Part model, mm, in its own coordinate system. Coordinates: 2 decimals unless noted, no trailing zeros. Order: outer loops, then holes, each group sorted by start corner. A loop starts at its lowest first (then second) coordinate and runs counter-clockwise, first axis right, second up.
from build123d import *

# Parameters (mm, degrees)
SKETCH1_R           = 2.413
SKETCH1_R_2         = 2.032
SKETCH1_R_3         = 7.9375
SKETCH1_R_4         = 3.175
BOSS_EXTRUDE1_DEPTH = 1.27
SKETCH2_R           = 2.413
CUT_EXTRUDE1_DEPTH  = 2.27
FILLET1_R           = 6.35


with BuildPart() as part:
    # Sketch1 → Boss-Extrude1 (new body)
    with BuildSketch(Plane.XY):
        with BuildLine():
            ThreePointArc((82.933641233, -259.730513994), (142.159112513, -114.876836591), (34.858765173, -0.960728132))
            ThreePointArc((34.858765173, -0.960728132), (26.627499814, 4.377145212), (23.4315, 13.6525))
            Line((23.4315, 13.6525), (23.4315, 42.2275))
            ThreePointArc((23.4315, 42.2275), (20.176724106, 50.085224106), (12.319, 53.34))
            Line((12.319, 53.34), (-12.319, 53.34))
            ThreePointArc((-12.319, 53.34), (-20.176724106, 50.085224106), (-23.4315, 42.2275))
            Line((-23.4315, 42.2275), (-23.4315, 13.6525))
            ThreePointArc((-23.4315, 13.6525), (-28.906938551, 6.162526908), (-37.733581796, 3.30411944))
            Line((-37.733581796, 3.30411944), (-164.5412, 3.30411944))
            ThreePointArc((-164.5412, 3.30411944), (-173.521456121, -0.415624439), (-177.2412, -9.39588056))
            Line((-177.2412, -9.39588056), (-177.2412, -41.275))
            ThreePointArc((-177.2412, -41.275), (-173.521456121, -50.255256121), (-164.5412, -53.975))
            ThreePointArc((-164.5412, -53.975), (-140.291720841, -66.502733348), (-136.476647403, -93.529138158))
            ThreePointArc((-136.476647403, -93.529138158), (-137.626098624, -185.624768634), (-82.933641233, -259.730513994))
            Line((-82.933641233, -259.730513994), (82.933641233, -259.730513994))
        make_face()
        with Locations((-96.602601281, -227.966886439)):
            Circle(SKETCH1_R, mode=Mode.SUBTRACT)
        with Locations((-74.605556024, -215.266886439)):
            Circle(SKETCH1_R, mode=Mode.SUBTRACT)
        with Locations((-123.367851281, -181.608113561)):
            Circle(SKETCH1_R, mode=Mode.SUBTRACT)
        with Locations((-101.370806024, -168.908113561)):
            Circle(SKETCH1_R, mode=Mode.SUBTRACT)
        with Locations((-54.988413477, -232.353774031)):
            Circle(SKETCH1_R_2, mode=Mode.SUBTRACT)
        with Locations((-43.989890849, -226.003774031)):
            Circle(SKETCH1_R_2, mode=Mode.SUBTRACT)
        with Locations((43.989890849, -226.003774031)):
            Circle(SKETCH1_R_2, mode=Mode.SUBTRACT)
        with Locations((54.988413477, -232.353774031)):
            Circle(SKETCH1_R_2, mode=Mode.SUBTRACT)
        with Locations((74.605556024, -215.266886439)):
            Circle(SKETCH1_R, mode=Mode.SUBTRACT)
        with Locations((96.602601281, -227.966886439)):
            Circle(SKETCH1_R, mode=Mode.SUBTRACT)
        with Locations((101.370806024, -168.908113561)):
            Circle(SKETCH1_R, mode=Mode.SUBTRACT)
        with Locations((123.367851281, -181.608113561)):
            Circle(SKETCH1_R, mode=Mode.SUBTRACT)
        with Locations((0, -141.2875)):
            Circle(SKETCH1_R_3, mode=Mode.SUBTRACT)
        with Locations((106.359913477, -143.375725969)):
            Circle(SKETCH1_R_2, mode=Mode.SUBTRACT)
        with Locations((95.361390849, -137.025725969)):
            Circle(SKETCH1_R_2, mode=Mode.SUBTRACT)
        with Locations((-65.4812, -36.5125)):
            Circle(SKETCH1_R, mode=Mode.SUBTRACT)
        with Locations((-26.76525, -39.6875)):
            Circle(SKETCH1_R, mode=Mode.SUBTRACT)
        with Locations((-65.4812, -17.4625)):
            Circle(SKETCH1_R, mode=Mode.SUBTRACT)
        with Locations((-26.76525, -14.2875)):
            Circle(SKETCH1_R, mode=Mode.SUBTRACT)
        with Locations((-12.319, 23.1775)):
            Circle(SKETCH1_R_4, mode=Mode.SUBTRACT)
        with Locations((-12.319, 42.2275)):
            Circle(SKETCH1_R_4, mode=Mode.SUBTRACT)
        with Locations((51.3715, -60.833)):
            Circle(SKETCH1_R_2, mode=Mode.SUBTRACT)
        with Locations((26.76525, -39.6875)):
            Circle(SKETCH1_R, mode=Mode.SUBTRACT)
        with Locations((51.3715, -48.133)):
            Circle(SKETCH1_R_2, mode=Mode.SUBTRACT)
        with Locations((26.76525, -14.2875)):
            Circle(SKETCH1_R, mode=Mode.SUBTRACT)
        with Locations((12.319, 23.1775)):
            Circle(SKETCH1_R_4, mode=Mode.SUBTRACT)
        with Locations((12.319, 42.2275)):
            Circle(SKETCH1_R_4, mode=Mode.SUBTRACT)
    extrude(amount=BOSS_EXTRUDE1_DEPTH)

    # Sketch2 → Cut-Extrude1 (cut, through all)
    with BuildSketch(Plane.XY.offset(1.27)):
        with Locations((-102.3112, -17.4625)):
            Circle(SKETCH2_R)
        with Locations((-102.3112, -36.5125)):
            Circle(SKETCH2_R)
    extrude(amount=-CUT_EXTRUDE1_DEPTH, mode=Mode.SUBTRACT)

    # Fillet1
    fillet1_edges = [part.edges().sort_by_distance(p)[0] for p in [
        (82.933641233, -259.730513994, 0.635),
        (-82.933641233, -259.730513994, 0.635),
    ]]
    fillet(fillet1_edges, radius=FILLET1_R)


solid = part.part
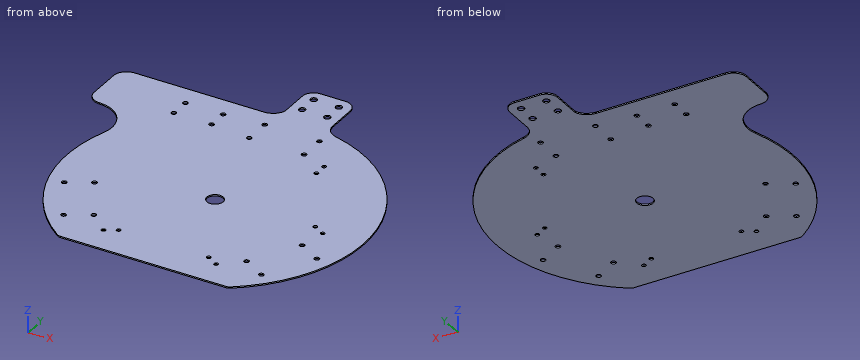
Q1. Cut at C-C on z = 0.35. Count the separate pieces of the cut face and the enclosed holes in it, and give its area (3 significant figures).
Results list:
separate pieces: 1
enclosed holes: 29
area: 70,400 mm2
Q2. Cut at A-A on x = 0. Write the cut outline in (y, z) (3 decimals), and give its area (3 significant figures).
Results list:
outline: (-259.731, 0) - (-149.225, 0) - (-149.225, 1.27) - (-259.731, 1.27) - close; (-133.35, 0) - (53.34, 0) - (53.34, 1.27) - (-133.35, 1.27) - close
area: 377 mm2
Q3. Wall check: line 1 along X through (y, z) = (-216, 0.3); line 2 along Y through (x, z) = (-75, 0.9); line 3 along Y through (x, z) = (52.5, 0.2). Give the ranges that are in metal, low to high.
Results list:
line 1: x = -123.79 to -76.9, -72.31 to 72.31, 76.9 to 123.79
line 2: y = -259.73 to -217.65, -212.89 to 3.3
line 3: y = -259.73 to -62.52, -59.14 to -49.82, -46.44 to -6.56
Q4. Cut at B-B on y = 33.5. Write the cut outline in (x, z).
Results list:
outline: (-23.43, 0) - (23.43, 0) - (23.43, 1.27) - (-23.43, 1.27) - close
